For this review, take the finished solid that the model builds, in its own axes (mm). A direction names the side the tool comes from. Coordinates: 2 decimals unless noted, no trailing zeros. Write each loop counter-clockwise with the first axis right and the second up, starting at its lowest first coordinate (ties: lowest second). Pieces come first, ordered by that corner, then holes. Notation, with made-up numbers: (59, 2) -> (96, 2) arc R9 ccw to (96, 19) -> close; hole circle Ø4 at (76, 28). An arc over 180 degrees is marked (long way). One line per item, written item: value. Start each with the question number.
1) Add section B-B (x = 8.5). State the section outline as (y, z) points.
2) Add section D-D (y = 0.45). State the section outline as (x, z) points (3 decimals), and give its area (3 significant figures).
3) Add section C-C (x = -14.5). State the section outline as (y, z) points.
4) Machinability: for faces 5 (the flat face through (-13, 1, 12.5)), 6 (the flat face through (-14, 1.5, 6)), 7 (the flat face through (-17, 1, 0)), which of the approach directions +Z, -Z, +X, -X, +Y, -Y give a long, thin tool a straight path to every point of the face, cutting with its end or side? Answer none if there is none.
5) For probe 1 along X at (y, z) = (0.8, 21) (3 decimals); probe 2 along Z at (x, y) = (-15, 0.45); probe 3 along Y at (x, z) = (14.6, -3.75), list the stretches that pass through material, from the lowest coordinate up. Write a range as from..to.
6) Add section A-A (z = -11). State the section outline as (x, y) points, and give its area (3 significant figures).
7) For pin 1 Ø1.1 at (x, z) = (8.5, -11) entering from +Y; pin 2 Ø3 at (x, z) = (-14.5, 7.37) entering from -Y; pin 3 Ø1.5 at (y, z) = (2.5, 14) entering from -X, all flat-tipped, find the tip position at first contact; note any pin that passes through.
8) Mouldability with a two-part tool opening along X and no side actions: class faces 1 (the flat face through (0, 1, -12.5)), 2 (the flat face through (17, 1, 5)), 3 (the cylindrical face through (-2.355, 2.24, 20.446)), 4 (the cylindrical face through (7.914, 2.24, -10.87)) as released by +X, released by -X, zero draft, split by the parting line, or undercut.
from build123d import *

# Parameters (mm, degrees)
EXTRUDE_1_DEPTH     = 3
SKETCH_2_R          = 1.25
SKETCH_2_R_2        = 0.6
CUT_EXTRUDE_1_DEPTH = 29.359301825
SKETCH_2_3_R        = 2
SKETCH_2_3_R_2      = 1
CUT_EXTRUDE_2_DEPTH = 1.5
SKETCH_3_R          = 0.35
CUT_EXTRUDE_3_DEPTH = 3


with BuildPart() as part:
    # Sketch 1 → Extrude 1 (new body)
    with BuildSketch(Plane(origin=(0, 0, 0), x_dir=(1, 0, 0), z_dir=(0, 1, 0))):
        Polygon((-17, 12.5), (-17, -12.5), (-8.5, -12.5), (-8.5, -22.5), (17, -22.5), (17, 12.5), align=None)
    extrude(amount=EXTRUDE_1_DEPTH)

    # Sketch 2 → Cut-Extrude 1 (cut, through all)
    with BuildSketch(Plane(origin=(0, 0, 0), x_dir=(-1, 0, 0), z_dir=(0, -1, 0))):
        with Locations(Location((14.499999998, -7.374985298, 0), (0, 0, 90))):
            Circle(SKETCH_2_R)
        with Locations(Location((14.499999998, 3.875014702, 0), (0, 0, 90))):
            Circle(SKETCH_2_R)
        with Locations(Location((-10.625, -21, 0), (0, 0, 90))):
            Circle(SKETCH_2_R_2)
        with Locations(Location((2.125, -21, 0), (0, 0, 90))):
            Circle(SKETCH_2_R_2)
        with Locations(Location((-8.5, 11, 0), (0, 0, 90))):
            Circle(SKETCH_2_R_2)
        with Locations(Location((8.5, 11, 0), (0, 0, 90))):
            Circle(SKETCH_2_R_2)
    extrude(amount=-CUT_EXTRUDE_1_DEPTH, mode=Mode.SUBTRACT)

    # Sketch 2_3 → Cut-Extrude 2 (cut)
    with BuildSketch(Plane(origin=(0, 0, 0), x_dir=(-1, 0, 0), z_dir=(0, -1, 0))):
        with Locations(Location((14.499999998, 3.875014702, 0), (0, 0, 90))):
            Circle(SKETCH_2_3_R)
        with Locations(Location((14.499999998, -7.374985298, 0), (0, 0, 90))):
            Circle(SKETCH_2_3_R)
        with Locations(Location((-10.625, -21, 0), (0, 0, 90))):
            Circle(SKETCH_2_3_R_2)
        with Locations(Location((2.125, -21, 0), (0, 0, 90))):
            Circle(SKETCH_2_3_R_2)
        with Locations(Location((-8.5, 11, 0), (0, 0, 90))):
            Circle(SKETCH_2_3_R_2)
        with Locations(Location((8.5, 11, 0), (0, 0, 90))):
            Circle(SKETCH_2_3_R_2)
    extrude(amount=-CUT_EXTRUDE_2_DEPTH, mode=Mode.SUBTRACT)

    # Sketch 3 → Cut-Extrude 3 (cut)
    with BuildSketch(Plane(origin=(17, 0, 0), x_dir=(0, 0, -1), z_dir=(1, 0, 0))):
        with Locations((3.75, 1.5)):
            Circle(SKETCH_3_R)
        with Locations((-13.75, 1.5)):
            Circle(SKETCH_3_R)
    extrude(amount=-CUT_EXTRUDE_3_DEPTH, mode=Mode.SUBTRACT)


solid = part.part
Numbers:
1. outline: (0, -12.5) -> (3, -12.5) -> (3, -11.6) -> (1.5, -11.6) -> (1.5, -12) -> (0, -12) -> close; (0, -10) -> (1.5, -10) -> (1.5, -10.4) -> (3, -10.4) -> (3, 22.5) -> (0, 22.5) -> close
2. outline: (-17, -12.5) -> (17, -12.5) -> (17, 22.5) -> (-8.5, 22.5) -> (-8.5, 12.5) -> (-17, 12.5) -> close; hole circle Ø4 at (-14.5, -3.875); hole circle Ø4 at (-14.5, 7.375); hole circle Ø2 at (-8.5, -11); hole circle Ø2 at (-2.125, 21); hole circle Ø2 at (8.5, -11); hole circle Ø2 at (10.625, 21)
2. area: 1,070 mm²
3. outline: (0, -12.5) -> (3, -12.5) -> (3, -5.13) -> (1.5, -5.13) -> (1.5, -5.88) -> (0, -5.88) -> close; (0, -1.88) -> (1.5, -1.88) -> (1.5, -2.63) -> (3, -2.63) -> (3, 6.12) -> (1.5, 6.12) -> (1.5, 5.37) -> (0, 5.37) -> close; (0, 9.37) -> (1.5, 9.37) -> (1.5, 8.62) -> (3, 8.62) -> (3, 12.5) -> (0, 12.5) -> close
4. face 5: +Z, -X, +Y, -Y
4. face 6: -Y
4. face 7: +Z, -Z, -X, +Y, -Y
5. probe 1: -8.5..-3.125, -1.125..9.625, 11.625..17
5. probe 2: -12.5..-5.81, -1.94..5.44, 9.31..12.5
5. probe 3: 0..1.15, 1.85..3
6. outline: (-17, 0) -> (-9.5, 0) -> (-9.5, 1.5) -> (-9.1, 1.5) -> (-9.1, 3) -> (-17, 3) -> close; (-7.9, 1.5) -> (-7.5, 1.5) -> (-7.5, 0) -> (7.5, 0) -> (7.5, 1.5) -> (7.9, 1.5) -> (7.9, 3) -> (-7.9, 3) -> close; (9.1, 1.5) -> (9.5, 1.5) -> (9.5, 0) -> (17, 0) -> (17, 3) -> (9.1, 3) -> close
6. area: 92.4 mm²
7. pin 1: through
7. pin 2: y = 1.5
7. pin 3: x = -8.5
8. face 1: zero draft
8. face 2: released by +X
8. face 3: undercut
8. face 4: undercut
